For this review, take the finished solid that the model builds, in its own axes (mm). Round coordinates to 2 decimals unless told otherwise and drop trailing zeros. Write each loop counter-clockwise with the first axis right and the second up, starting at its lowest first coordinate (ties: lowest second). Pieces come first, ordered by that corner, then holes. Notation, with made-up numbers: (-13, 50.25) -> (33, 50.25) arc R28 ccw to (33, 83.25) -> close; hole circle Ø5 at (-37, 76.5). An arc over 180 degrees is marked (long way). Write item = value, one per line. Start each with the question number.
```python
from build123d import *

# Parameters (mm, degrees)
SKETCH8_R           = 1.075
BOSS_EXTRUDE1_DEPTH = 1.15


with BuildPart() as part:
    # Sketch6 → Revolve-Thin2 (revolve)
    with BuildSketch(Plane(origin=(0, 0, 0), x_dir=(0, 0, -1), z_dir=(1, 0, 0))):
        with BuildLine():
            Line((-3.75, 0), (-3.75, 2))
            ThreePointArc((-3.75, 2), (-3.632270634, 2.403402832), (-3.31604308, 2.680159372))
            Line((-3.31604308, 2.680159372), (-1.50895692, 3.519840628))
            ThreePointArc((-1.50895692, 3.519840628), (-1.192729366, 3.796597168), (-1.075, 4.2))
            Line((-1.075, 4.2), (-1.075, 6.2))
            Line((-1.075, 6.2), (-0.425, 6.2))
            Line((-0.425, 6.2), (-0.425, 4.2))
            ThreePointArc((-0.425, 4.2), (-0.644761483, 3.44698138), (-1.235052917, 2.930369172))
            Line((-1.235052917, 2.930369172), (-3.042139077, 2.090687916))
            ThreePointArc((-3.042139077, 2.090687916), (-3.084302751, 2.053787044), (-3.1, 2))
            Line((-3.1, 2), (-3.1, 0))
            Line((-3.1, 0), (-3.75, 0))
        make_face()
    revolve(axis=Axis((0, -0.227579974, 0), (0, 1, 0)))

    # Sketch8 → Boss-Extrude1 (add)
    with BuildSketch(Plane(origin=(0, 6.2, 0), x_dir=(1, 0, 0), z_dir=(0, 1, 0))):
        Circle(SKETCH8_R)
    extrude(amount=BOSS_EXTRUDE1_DEPTH)


solid = part.part
```
1. Wall thickness on L1, parallel to X at y = 5, z = 0 (3 decimals); L2, parallel to X at y = 0.75, z = 0; L3, parallel to X at y = 7.25, z = 0 (3 decimals): over which ranges is each line inside the solid? List them lowest first. Write a range as from..to.
2. Consider section D-D, the plane y = 1.75. Give the boundary of the cut face in (x, z), then the cut area to 3 significant figures.
3. Consider section C-C, the plane y = 4.5. Give the boundary of the cut face in (x, z) (3 decimals), then the cut area to 3 significant figures.
4. Draft analysis for pull direction Z (two halves, no side actions). For faces 1 (the cylindrical face through (0.165, 1.014, -3.746)), 2 (the cylindrical face through (-2.75, 0.99, 1.43)), 3 (the flat face through (0, 7.35, 0)), state which applies: +Z half, -Z half, draft (parallel to the pull), parting line (faces both ways), or undercut.
5. Consider section A-A, the plane z = 0. Give the boundary of the cut face in (x, y) (3 decimals).
6. Clearance check with flat-ended pins moving along their axes: pin 1 Ø1.5 at (x, y) = (1.5, 2.5) entering from -Z; pin 2 Ø1.5 at (y, z) = (1.5, -1) entering from +X; pin 3 Ø1.5 at (x, y) = (1, 1) entering from -Z. State where each tip first meets the part, or that it passes through.
7. Consider section B-B, the plane x = 0. Give the boundary of the cut face in (y, z) (3 decimals).
Outcome:
q1.L1 = -1.075..-0.425, 0.425..1.075
q1.L2 = -3.75..-3.1, 3.1..3.75
q1.L3 = -1.075..1.075
q2.outline = circle Ø7.5 at (0, 0); hole circle Ø6.2 at (0, 0)
q2.area = 14.0 mm2
q3.outline = circle Ø2.15 at (0, 0); hole circle Ø0.85 at (0, 0)
q3.area = 3.06 mm2
q4.face_1 = parting line
q4.face_2 = undercut
q4.face_3 = draft
q5.outline = (-3.75, 0) -> (-3.1, 0) -> (-3.1, 2) arc R0.1 cw to (-3.042, 2.091) -> (-1.235, 2.93) arc R1.4 ccw to (-0.425, 4.2) -> (-0.425, 6.2) -> (0.425, 6.2) -> (0.425, 4.2) arc R1.4 ccw to (1.235, 2.93) -> (3.042, 2.091) arc R0.1 cw to (3.1, 2) -> (3.1, 0) -> (3.75, 0) -> (3.75, 2) arc R0.75 ccw to (3.316, 2.68) -> (1.509, 3.52) arc R0.75 cw to (1.075, 4.2) -> (1.075, 7.35) -> (-1.075, 7.35) -> (-1.075, 4.2) arc R0.75 cw to (-1.509, 3.52) -> (-3.316, 2.68) arc R0.75 ccw to (-3.75, 2) -> close
q6.pin_1 = -3.64
q6.pin_2 = 3.74
q6.pin_3 = -3.74
q7.outline = (0, -3.75) -> (2, -3.75) arc R0.75 ccw to (2.68, -3.316) -> (3.52, -1.509) arc R0.75 cw to (4.2, -1.075) -> (7.35, -1.075) -> (7.35, 1.075) -> (4.2, 1.075) arc R0.75 cw to (3.52, 1.509) -> (2.68, 3.316) arc R0.75 ccw to (2, 3.75) -> (0, 3.75) -> (0, 3.1) -> (2, 3.1) arc R0.1 cw to (2.091, 3.042) -> (2.93, 1.235) arc R1.4 ccw to (4.2, 0.425) -> (6.2, 0.425) -> (6.2, -0.425) -> (4.2, -0.425) arc R1.4 ccw to (2.93, -1.235) -> (2.091, -3.042) arc R0.1 cw to (2, -3.1) -> (0, -3.1) -> close
